Part print with two shaded views. Sizes in mm from the minimum x, y, z corner. Round coordinates to 2 decimals unless told otherwise and drop trailing zeros. Write each loop counter-clockwise with the first axis right and the second up, starting at its lowest first coordinate (ties: lowest second). Pieces come first, ordered by that corner, then holes. Notation, with made-up numbers: (16, -5) -> (71, -5) arc R20 cw to (71, 31) -> close; hole circle Ø5 at (88.5, 18.5). An arc over 180 degrees is marked (long way). Answer in a Markdown table with one row per item.
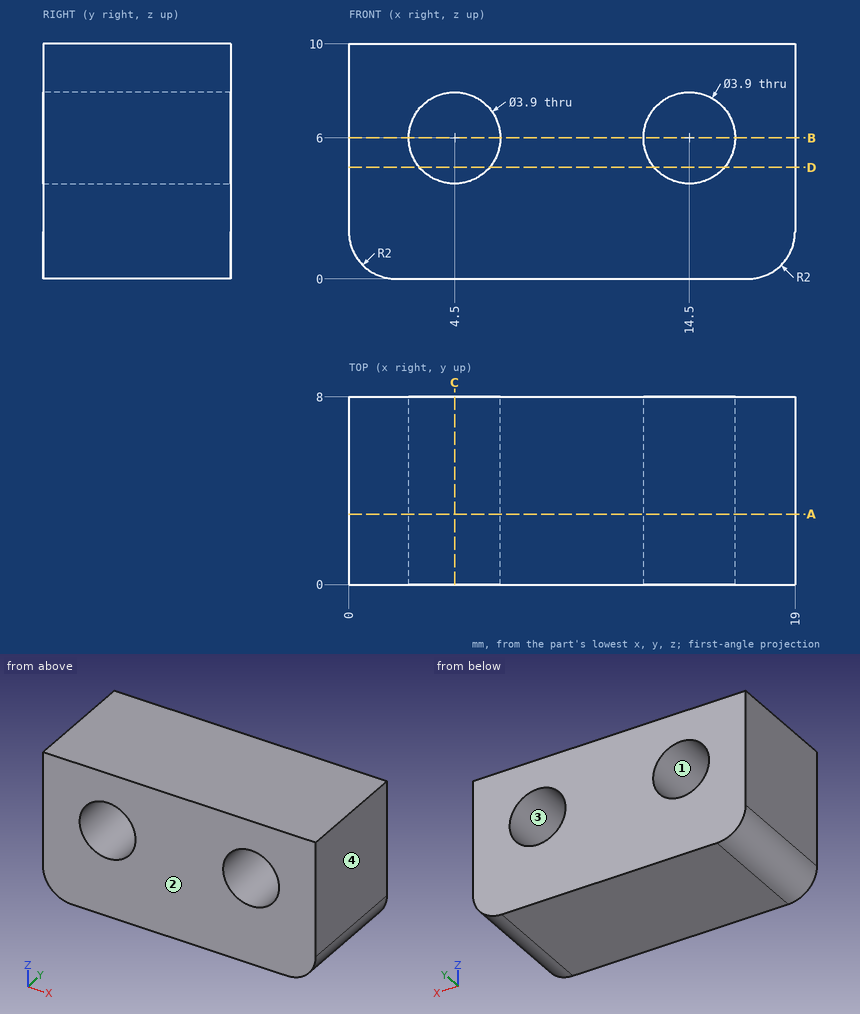
Q1. Saw through at C-C on x = 4.5. Write the cut outline in (y, z), plus the area to 3 significant figures.
A:
| item | result |
|---|---|
| outline | (0, 0) -> (8, 0) -> (8, 4.05) -> (0, 4.05) -> close; (0, 7.95) -> (8, 7.95) -> (8, 10) -> (0, 10) -> close |
| area | 48.8 mm² |
Q2. Saw through at D-D on z = 4.75. Write the cut outline in (x, y).
A:
| item | result |
|---|---|
| outline | (0, 0) -> (3, 0) -> (3, 8) -> (0, 8) -> close; (6, 0) -> (13, 0) -> (13, 8) -> (6, 8) -> close; (16, 0) -> (19, 0) -> (19, 8) -> (16, 8) -> close |
Q3. Two-plate mould, pull along X, no slides. Class the marked faces 1, 2, 3 and 4: released by +X, released by -X, zero draft, split by the parting line, or undercut.
A:
| item | result |
|---|---|
| face 1 | undercut |
| face 2 | zero draft |
| face 3 | undercut |
| face 4 | released by +X |
Q4. Wall check: line 1 (X direction, y = 6, z = 6); line 2 (X direction, y = 0.5, z = 4.5); line 3 (Z direction, x = 15.5, y = 4.75). Give the ranges that are in metal, low to high. Write a range as [from, to].
A:
| item | result |
|---|---|
| line 1 | [0, 2.55], [6.45, 12.55], [16.45, 19] |
| line 2 | [0, 3.25], [5.75, 13.25], [15.75, 19] |
| line 3 | [0, 4.33], [7.67, 10] |
Q5. Saw through at B-B on z = 6. Write the cut outline in (x, y), plus the area to 3 significant figures.
A:
| item | result |
|---|---|
| outline | (0, 0) -> (2.55, 0) -> (2.55, 8) -> (0, 8) -> close; (6.45, 0) -> (12.55, 0) -> (12.55, 8) -> (6.45, 8) -> close; (16.45, 0) -> (19, 0) -> (19, 8) -> (16.45, 8) -> close |
| area | 89.6 mm² |
Q6. Drop a flat-ended pin along its axis: P1, Ø2.5, axis at x = 14.5, z = 6, coming from the -Y side. Give the stop position or say it passes through.
A:
| item | result |
|---|---|
| P1 | through |
Q7. Saw through at A-A on y = 3. Write the cut outline in (x, z).
A:
| item | result |
|---|---|
| outline | (0, 2) arc R2 ccw to (2, 0) -> (17, 0) arc R2 ccw to (19, 2) -> (19, 10) -> (0, 10) -> close; hole circle Ø3.9 at (4.5, 6); hole circle Ø3.9 at (14.5, 6) |
